from build123d import *

# Parameters (mm, degrees)
F0_R     = 57.85
F0_R_2   = 22.5
F1_DEPTH = 6
F2_R     = 57.85
F2_R_2   = 55.35
F3_DEPTH = 3


with BuildPart() as f1:
    # F0 (on Front) → F1 (new body)
    with BuildSketch(Plane.XZ):
        Circle(F0_R)
        with BuildLine():
            ThreePointArc((-12.320414, -37.950196), (-10.329128, -41.855933), (-14.234864, -43.847219))
            ThreePointArc((-14.234864, -43.847219), (-23.05, -39.923771), (-30.855373, -34.251364))
            ThreePointArc((-30.855373, -34.251364), (-31.083737, -29.873254), (-26.705627, -29.64489))
            ThreePointArc((-26.705627, -29.64489), (-19.95, -34.554414), (-12.320414, -37.950196))
        make_face(mode=Mode.SUBTRACT)
        with BuildLine():
            ThreePointArc((-27.372431, 15.803481), (-25.159068, 13.141948), (-25.204864, 9.680642))
            ThreePointArc((-25.204864, 9.680642), (-27, 0), (-25.204864, -9.680642))
            ThreePointArc((-25.204864, -9.680642), (-25.159068, -13.141948), (-27.372431, -15.803481))
            Line((-27.372431, -15.803481), (-38.729833, -22.36068))
            ThreePointArc((-38.729833, -22.36068), (-42.790653, -22.780694), (-45.810926, -20.033948))
            ThreePointArc((-45.810926, -20.033948), (-50, 0), (-45.810926, 20.033948))
            ThreePointArc((-45.810926, 20.033948), (-42.790653, 22.780694), (-38.729833, 22.36068))
            Line((-38.729833, 22.36068), (-27.372431, 15.803481))
        make_face(mode=Mode.SUBTRACT)
        Circle(F0_R_2, mode=Mode.SUBTRACT)
        with BuildLine():
            Line((0, -44.72136), (0, -31.606961))
            ThreePointArc((0, -31.606961), (1.198273, -28.359366), (4.21875, -26.668374))
            ThreePointArc((4.21875, -26.668374), (13.5, -23.382686), (20.986114, -16.987731))
            ThreePointArc((20.986114, -16.987731), (23.960795, -15.217418), (27.372431, -15.803481))
            Line((27.372431, -15.803481), (38.729833, -22.36068))
            ThreePointArc((38.729833, -22.36068), (41.123986, -25.667445), (40.255371, -29.656452))
            ThreePointArc((40.255371, -29.656452), (25, -43.30127), (5.555556, -49.690399))
            ThreePointArc((5.555556, -49.690399), (1.666667, -48.44814), (0, -44.72136))
        make_face(mode=Mode.SUBTRACT)
        with BuildLine():
            ThreePointArc((45.090238, 9.595855), (46.1, 0), (45.090238, -9.595855))
            ThreePointArc((45.090238, -9.595855), (41.412865, -11.982679), (39.026041, -8.305306))
            ThreePointArc((39.026041, -8.305306), (39.9, 0), (39.026041, 8.305306))
            ThreePointArc((39.026041, 8.305306), (41.412865, 11.982679), (45.090238, 9.595855))
        make_face(mode=Mode.SUBTRACT)
        with BuildLine():
            ThreePointArc((-30.855373, 34.251364), (-23.05, 39.923771), (-14.234864, 43.847219))
            ThreePointArc((-14.234864, 43.847219), (-10.329128, 41.855933), (-12.320414, 37.950196))
            ThreePointArc((-12.320414, 37.950196), (-19.95, 34.554414), (-26.705627, 29.64489))
            ThreePointArc((-26.705627, 29.64489), (-31.083737, 29.873254), (-30.855373, 34.251364))
        make_face(mode=Mode.SUBTRACT)
        with BuildLine():
            ThreePointArc((20.986114, 16.987731), (13.5, 23.382686), (4.21875, 26.668374))
            ThreePointArc((4.21875, 26.668374), (1.198273, 28.359366), (0, 31.606961))
            Line((0, 31.606961), (0, 44.72136))
            ThreePointArc((0, 44.72136), (1.666667, 48.44814), (5.555556, 49.690399))
            ThreePointArc((5.555556, 49.690399), (25, 43.30127), (40.255371, 29.656452))
            ThreePointArc((40.255371, 29.656452), (41.123986, 25.667445), (38.729833, 22.36068))
            Line((38.729833, 22.36068), (27.372431, 15.803481))
            ThreePointArc((27.372431, 15.803481), (23.960795, 15.217418), (20.986114, 16.987731))
        make_face(mode=Mode.SUBTRACT)
    extrude(amount=F1_DEPTH)

    # F2 (on face) → F3 (cut)
    with BuildSketch(Plane(origin=(0, 0, 0), x_dir=(-1, 0, 0), z_dir=(0, 1, 0))):
        Circle(F2_R)
        Circle(F2_R_2, mode=Mode.SUBTRACT)
    extrude(amount=-F3_DEPTH, mode=Mode.SUBTRACT)


solid = f1.part
The model under review builds one solid part; all positions refer to its coordinate system, in mm. A direction names the side the tool comes from. Give positions to 0.01 mm unless a question says otherwise; leave off trailing zeros. Write each loop counter-clockwise with the first axis right and the second up, starting at its lowest first coordinate (ties: lowest second). Pieces come first, ordered by that corner, then holes. Notation, with made-up numbers: M 38,37.25 L 74,37.25 A12 cw 74,48.25 Z; hole C 70.25,70.25 d3. An arc over 180 degrees is marked long. One line per question, with ' | ' between items. Start each with the question number.
Item 1: We need section D-D on y = -1.85. Give the number of separate pieces and of enclosed holes in the cut face, plus the area to 3 significant figures.
Item 2: Wall thickness on line 1 (X direction, y = -0.95, z = -20.5); line 2 (X direction, y = -1.3, z = -34.5); line 3 (Z direction, x = -17, y = -1.05): over which ranges is each line inside the solid? List them lowest first. Write a range as from..to.
Item 3: For pin 1 (1.5 mm diameter, centred on y = -3, z = 22, fed in from +X); pin 2 (2 mm diameter, centred on x = -27.5, y = -1.5, fed in from +Z); pin 3 (1.8 mm diameter, centred on y = -2.5, z = -40, fed in from +X); pin 4 (3 mm diameter, centred on x = -38, z = 27.5, fed in from +Y), all flat-tipped, find the tip position at first contact; note any pin that passes through.
Item 4: We need section C-C on x = 34.5. Write out the cut boundary in (y, z).
Item 5: For faces 1 (the flat face through (-32.972, -2.958, -19.036)), 2 (the flat face through (-1, -6, -25)), list the 3-axis set-ups (+Z, -Z, +X, -X, +Y, -Y) from which the entire face can be reached by the end or side of a thin tool; tool diameter is ignored.
Item 6: We need section A-A on z = 0. Write out the cut boundary in (x, y).
Item 7: We need section B-B on x = -8.5. Write out the cut boundary in (y, z).
Item 8: Draft analysis for pull direction X (two halves, no side actions). For faces 3 (the cylindrical face through (-25.143, -2.958, -13.095)), 4 (the flat face through (-30, -3, -47)), state which applies: released by +X, released by -X, zero draft, split by the parting line, or undercut.
Results found:
1) separate pieces: 1 | enclosed holes: 7 | area: 4,890 mm2
2) line 1: x = -51.41..-45.58, -35.51..-9.27, 9.27..17.57, 35.51..51.41 | line 2: x = -43.28..-30.58, -20.04..0, 36.19..43.28 | line 3: z = -52.67..-42.85, -36.1..-14.74, 14.74..36.1, 42.85..52.67
3) pin 1: stops at x = 53.81 | pin 2: stops at z = 48.59 | pin 3: stops at x = 42.5 | pin 4: stops at y = 0
4) outline: M -6,-46.44 L -3,-46.44 L -3,-43.28 L 0,-43.28 L 0,-36.19 L -6,-36.19 Z; M -6,-19.92 L 0,-19.92 L 0,19.92 L -6,19.92 Z; M -6,36.19 L 0,36.19 L 0,43.28 L -3,43.28 L -3,46.44 L -6,46.44 Z
5) face 1: +Y, -Y | face 2: +Z, -Z, +X, -X, -Y
6) outline: M -57.85,-6 L -50,-6 L -50,0 L -55.35,0 L -55.35,-3 L -57.85,-3 Z; M -27,-6 L -22.5,-6 L -22.5,0 L -27,0 Z; M 22.5,-6 L 39.9,-6 L 39.9,0 L 22.5,0 Z; M 46.1,-6 L 57.85,-6 L 57.85,-3 L 55.35,-3 L 55.35,0 L 46.1,0 Z
7) outline: M -6,-57.22 L -3,-57.22 L -3,-54.69 L 0,-54.69 L 0,-20.83 L -6,-20.83 Z; M -6,20.83 L 0,20.83 L 0,54.69 L -3,54.69 L -3,57.22 L -6,57.22 Z
8) face 3: undercut | face 4: zero draft
